```python
from build123d import *

# Parameters (mm, degrees)
F0_R     = 12.95
F1_DEPTH = 3


with BuildPart() as f1:
    # F0 (on Top) → F1 (new body)
    with BuildSketch(Plane.XY):
        with BuildLine():
            Line((-22, -15), (22, -15))
            ThreePointArc((22, -15), (47, 0), (22, 15))
            Line((22, 15), (-22, 15))
            ThreePointArc((-22, 15), (-47, 0), (-22, -15))
        make_face()
        with Locations((-30, 0)):
            Circle(F0_R, mode=Mode.SUBTRACT)
        with BuildLine():
            ThreePointArc((0, 11), (11, 0), (0, -11))
            ThreePointArc((0, -11), (-11, 0), (0, 11))
        make_face(mode=Mode.SUBTRACT)
        with Locations((30, 0)):
            Circle(F0_R, mode=Mode.SUBTRACT)
    extrude(amount=F1_DEPTH)


solid = f1.part
```
Model file for the job. Use its own axes, mm. A direction names the side the tool comes from. Coordinates: 2 decimals unless noted, no trailing zeros. Order: outer loops, then holes, each group sorted by start corner. A loop starts at its lowest first (then second) coordinate and runs counter-clockwise, first axis right, second up. Notation, with made-up numbers: (22, 35.25) -> (42, 35.25) arc R25 cw to (42, 48.25) -> close; hole circle Ø1 at (-38, 20.5). An arc over 180 degrees is marked (long way). Answer as a JSON object with one key per item and string values. Group by question number.
1) Cut at C-C, the plane z = 2. Write the cut outline in (x, y).
2) Drill centre lines: L1, parallel to Y at x = 30, z = 0.8; L2, parallel to Y at x = 0, z = 2; L3, parallel to X at y = 8.5, z = 1.3. Where is each one in solid material? Low to high.
3) Cut at B-B, the plane y = 0. Write the cut outline in (x, z), then the cut area to 3 significant figures.
4) Flat gauge pins, fed straight in: pin 1 (1 mm diameter, centred on y = -2.5, z = 0.5, fed in from +X); pin 2 (5 mm diameter, centred on x = 29.5, y = -10.5, fed in from -Z); pin 3 (0.9 mm diameter, centred on x = -7, z = 1.5, fed in from -Y); pin 4 (15.5 mm diameter, centred on x = -30, y = 0, fed in from +Z). Where does each tip first touch, or does it go through?
5) Pull direction Y, two halves, no side cores. Call faces 1 (the face through (-42.937, 0.569, 1.479)), 2 (the face through (0, -15, 1)), 3 (the face through (-47, 0, 1)): +Y half, -Y half, draft (parallel to the pull), parting line (faces both ways), or undercut.
6) Cut at D-D, the plane x = 0. Write the cut outline in (y, z), then the cut area to 3 significant figures.
7) Which spindle directions (+Z, -Z, +X, -X, +Y, -Y) get a long thin tool onto all of the face, cutting with end or side? Do faces 4 (the face through (47, 0, 1)), 5 (the face through (0, 15, 1)). Say none if no direction does.
8) Cut at A-A, the plane x = 30. Write the cut outline in (y, z), then the cut area to 3 significant figures.
Check values:
{
 "1": {"outline": "(-22, -15) -> (22, -15) arc R17 ccw (long way) to (22, 15) -> (-22, 15) arc R17 ccw (long way) to start; hole circle Ø25.9 at (-30, 0); hole circle Ø22 at (0, 0); hole circle Ø25.9 at (30, 0)"},
 "2": {"L1": "y = -17 to -12.95, 12.95 to 17", "L2": "y = -15 to -11, 11 to 15", "L3": "x = -44.72 to -39.77, -20.23 to -6.98, 6.98 to 20.23, 39.77 to 44.72"},
 "3": {"outline": "(-47, 0) -> (-42.95, 0) -> (-42.95, 3) -> (-47, 3) -> close; (-17.05, 0) -> (-11, 0) -> (-11, 3) -> (-17.05, 3) -> close; (11, 0) -> (17.05, 0) -> (17.05, 3) -> (11, 3) -> close; (42.95, 0) -> (47, 0) -> (47, 3) -> (42.95, 3) -> close", "area": "60.6 mm²"},
 "4": {"pin 1": "stops at x = 46.88", "pin 2": "stops at z = 0", "pin 3": "stops at y = -15", "pin 4": "passes through"},
 "5": {"face 1": "undercut", "face 2": "-Y half", "face 3": "parting line"},
 "6": {"outline": "(-15, 0) -> (-11, 0) -> (-11, 3) -> (-15, 3) -> close; (11, 0) -> (15, 0) -> (15, 3) -> (11, 3) -> close", "area": "24.0 mm²"},
 "7": {"face 4": "+Z, -Z", "face 5": "+Z, -Z, +Y"},
 "8": {"outline": "(-17, 0) -> (-12.95, 0) -> (-12.95, 3) -> (-17, 3) -> close; (12.95, 0) -> (17, 0) -> (17, 3) -> (12.95, 3) -> close", "area": "24.3 mm²"}
}
